from build123d import *

# Parameters (mm, degrees)
ESQUISSE1_W        = 10
ESQUISSE1_H        = 60
BOSS_EXTRU_1_DEPTH = 4


with BuildPart() as part:
    # Esquisse1 → Boss.-Extru.1 (new body)
    with BuildSketch(Plane.XY):
        with BuildLine():
            Line((-5, 30), (5, 30))
            ThreePointArc((5, 30), (6.258850628, 44.9603643), (10, 59.5))
            Line((10, 59.5), (10, 75))
            Line((10, 75), (-10, 75))
            Line((-10, 75), (-10, 59.5))
            ThreePointArc((-10, 59.5), (-6.258850628, 44.9603643), (-5, 30))
        make_face()
        Rectangle(ESQUISSE1_W, ESQUISSE1_H)
        with BuildLine():
            Line((10, -59.5), (10, -75))
            Line((10, -75), (-10, -75))
            Line((-10, -75), (-10, -59.5))
            ThreePointArc((-10, -59.5), (-6.258850628, -44.9603643), (-5, -30))
            Line((-5, -30), (5, -30))
            ThreePointArc((5, -30), (6.258850628, -44.9603643), (10, -59.5))
        make_face()
    extrude(amount=BOSS_EXTRU_1_DEPTH)


solid = part.part
Geometry: final body of the model. Coordinates: model frame, mm. A direction names the side the tool comes from. Round coordinates to 2 decimals unless told otherwise and drop trailing zeros. Loops run counter-clockwise (first coordinate to the right, second up) from the corner with the lowest first, then second, coordinate; pieces in that order, holes last. Notation, with made-up numbers: (40.5, 19) - (46.5, 19) arc R25 ccw to (46.5, 45) - close; hole circle Ø7 at (15.5, -24). An arc over 180 degrees is marked (long way). Write each question's results on one line, items separated by ' | '. Start each with the question number.
1) Line query: probe 1 along X at (y, z) = (14, 0.75); probe 2 along X at (y, z) = (-52, 2.7). Output: solid intervals per line, ascending. Write a range as [from, to].
2) Mould query, pull axis Y, two halves, no side actions, for faces 1 (the face through (5, 0, 2)), 2 (the face through (0, 1, 0)), 3 (the face through (0, -75, 2)). Classes: released by +Y, released by -Y, zero draft, split by the parting line, or undercut.
3) Cut plane D-D on y = -44. Return loops of the section in (x, z), then the cut area to 3 significant figures.
4) Cut plane B-B on z = 3.3. Return loops of the section in (x, y) (3 decimals).
5) Cut plane C-C on y = -6. Return loops of the section in (x, z), then the cut area to 3 significant figures.
6) Cut plane A-A on x = -7.5. Return loops of the section in (y, z).
7) First-contact query: P1, Ø2, axis at y = 46.5, z = 2, coming from the +X side; P2, Ø1.2, axis at y = 1.5, z = 2.5, coming from the +X side. Flat tips, straight axial feed; report the tip coordinate or a pass-through.
8) Access query for faces 4 (the face through (-6.3, -45.2, 2)), 5 (the face through (6.224, -44.753, 1.972)), 6 (the face through (10, -67, 2)). Directions: +Z, -Z, +X, -X, +Y, -Y. A direction counts if a zero-diameter tool reaches every point of the face in a straight line with its end or side. Return the directions, or none.
Verdict:
1) probe 1: x = [-5, 5] | probe 2: x = [-7.75, 7.75]
2) face 1: undercut | face 2: zero draft | face 3: released by -Y
3) outline: (-6.1, 0) - (6.1, 0) - (6.1, 4) - (-6.1, 4) - close | area: 48.8 mm2
4) outline: (-10, -75) - (10, -75) - (10, -59.5) arc R89.525 cw to (5, -30) - (5, 30) arc R89.525 cw to (10, 59.5) - (10, 75) - (-10, 75) - (-10, 59.5) arc R89.525 cw to (-5, 30) - (-5, -30) arc R89.525 cw to (-10, -59.5) - close
5) outline: (-5, 0) - (5, 0) - (5, 4) - (-5, 4) - close | area: 40.0 mm2
6) outline: (-75, 0) - (-51.01, 0) - (-51.01, 4) - (-75, 4) - close; (51.01, 0) - (75, 0) - (75, 4) - (51.01, 4) - close
7) P1: stops at x = 6.73 | P2: stops at x = 5
8) face 4: +Z, -Z, -X | face 5: +Z, -Z, +X | face 6: +Z, -Z, +X, +Y, -Y
